Verification items for the finished model (mm, model axes). A direction names the side the tool comes from. Coordinates: 2 decimals unless noted, no trailing zeros. Write each loop counter-clockwise with the first axis right and the second up, starting at its lowest first coordinate (ties: lowest second). Pieces come first, ordered by that corner, then holes. Notation, with made-up numbers: (-32.75, -8) -> (-2.75, -8) arc R24 ccw to (-2.75, 12) -> close; hole circle Ø5 at (14, -4). An arc over 180 degrees is marked (long way). Answer in a Markdown table with one row per item.
```python
from build123d import *

# Parameters (mm, degrees)
F1_DEPTH  = 7.8
F2_R      = 6.44999
F3_R      = 2.7
F4_DEPTH  = 7.801
F5_R      = 4.2
F5_R_2    = 4.7163688055
F6_DEPTH  = 5.3
F8_DEPTH  = 10
F10_DEPTH = 5.2
F12_DEPTH = 9.8
F13_R     = 5
F14_R     = 7
F15_R     = 3
F16_R     = 3


# Not quite as in the source:
# - a fillet or chamfer is up to 0.001 mm smaller than in the source, because OpenCascade refuses the exact size


with BuildPart() as f1:
    # F0 (on Top) → F1 (new body)
    with BuildSketch(Plane.XY):
        Polygon((0, 68), (0, 12.9), (-10.05, 12.9), (-10.05, 0), (0, 0), (122, 0), (132.05, 0), (132.05, 12.9), (122, 12.9), (122, 58), (132.05, 58), (132.05, 70.9), (122, 70.9), (122, 87.4), (93.5, 87.4), (60, 68), (22.4718242228, 68), (22.4718242228, 78.05), (9.5718242228, 78.05), (9.5718242228, 68), align=None)
    extrude(amount=F1_DEPTH)

    # F2 (radius 6.45 in the source; OpenCascade refuses exactly that, so slightly less here)
    f2_edges = [f1.edges().sort_by_distance(p)[0] for p in [
        (-10.05, 0, 3.9),
        (-10.05, 12.9, 3.9),
        (9.571824, 78.05, 3.9),
        (22.471824, 78.05, 3.9),
        (132.05, 70.9, 3.9),
        (132.05, 58, 3.9),
        (132.05, 12.9, 3.9),
        (132.05, 0, 3.9),
    ]]
    fillet(f2_edges, radius=F2_R)

    # F3 (on face) → F4 (cut, through all)
    with BuildSketch(Plane.XY.offset(7.8)):
        with Locations((-3.6, 6.45)):
            Circle(F3_R)
        with Locations((16.0218242228, 71.6)):
            Circle(F3_R)
        with Locations((125.6, 64.45)):
            Circle(F3_R)
        with Locations((125.6, 6.45)):
            Circle(F3_R)
    extrude(amount=-F4_DEPTH, mode=Mode.SUBTRACT)

    # F5 (on face) → F6 (cut)
    with BuildSketch(Plane.XY.offset(7.8)):
        with Locations((-3.6, 6.45)):
            Circle(F5_R)
        with Locations((16.0218242228, 71.6)):
            Circle(F5_R)
        with Locations((125.6, 64.45)):
            Circle(F5_R_2)
        with Locations((125.6, 6.45)):
            Circle(F5_R_2)
    extrude(amount=-F6_DEPTH, mode=Mode.SUBTRACT)

    # F7 (on face) → F8 (join)
    with BuildSketch(Plane.XY.offset(7.8)):
        Polygon((5.3, 62.7), (5.3, 5.3), (116.7, 5.3), (116.7, 82.1), (94.9238653477, 82.1), (61.4238653477, 62.7), align=None)
    extrude(amount=F8_DEPTH)

    # F9 (on face) → F10 (cut)
    with BuildSketch(Plane(origin=(0, 0, 0), x_dir=(1, 0, 0), z_dir=(0, 0, -1))):
        Polygon((94.0910384462, -85.2), (119.8, -85.2), (119.8, -2.2), (2.2, -2.2), (2.2, -65.8), (60.5910384462, -65.8), align=None)
    extrude(amount=-F10_DEPTH, mode=Mode.SUBTRACT)

    # F11 (on face) → F12 (cut)
    with BuildSketch(Plane(origin=(0, 0, 5.2), x_dir=(1, 0, 0), z_dir=(0, 0, -1))):
        Polygon((114.5, -7.5), (7.5, -7.5), (7.5, -60.5), (62.0149037939, -60.5), (95.5149037939, -79.9), (114.5, -79.9), align=None)
    extrude(amount=-F12_DEPTH, mode=Mode.SUBTRACT)

    # F13
    f13_edges = [f1.edges().sort_by_distance(p)[0] for p in [
        (114.5, 79.9, 10.1),
        (119.8, 85.2, 2.6),
        (7.5, 60.5, 10.1),
        (2.2, 65.8, 2.6),
        (114.5, 7.5, 10.1),
        (7.5, 7.5, 10.1),
        (95.514904, 79.9, 10.1),
        (62.014904, 60.5, 10.1),
        (60.591038, 65.8, 2.6),
        (94.091038, 85.2, 2.6),
    ]]
    fillet(f13_edges, radius=F13_R)

    # F14
    f14_edges = [f1.edges().sort_by_distance(p)[0] for p in [
        (122, 87.4, 3.9),
        (93.5, 87.4, 3.9),
        (60, 68, 3.9),
        (61.423865, 62.7, 12.8),
        (94.923865, 82.1, 12.8),
        (116.7, 82.1, 12.8),
        (116.7, 5.3, 12.8),
        (5.3, 5.3, 12.8),
        (5.3, 62.7, 12.8),
        (0, 68, 3.9),
    ]]
    fillet(f14_edges, radius=F14_R)

    # F15
    f15_edges = [f1.edges().sort_by_distance(p)[0] for p in [
        (119.8, 2.2, 2.6),
        (2.2, 2.2, 2.6),
    ]]
    fillet(f15_edges, radius=F15_R)

    # F16
    f16_edges = [f1.edges().sort_by_distance(p)[0] for p in [
        (0, 12.9, 3.9),
        (9.571824, 68, 3.9),
        (22.471824, 68, 3.9),
        (122, 70.9, 3.9),
        (122, 58, 3.9),
        (122, 12.9, 3.9),
    ]]
    fillet(f16_edges, radius=F16_R)


solid = f1.part
```
1. Section check B-B, the plane x = 107. Record the boundary of the cut face in (y, z), plus the area to 3 significant figures.
Geometry says:
| item | result |
|---|---|
| outline | (0, 0) -> (2.2, 0) -> (2.2, 5.2) -> (7.5, 5.2) -> (7.5, 15) -> (79.9, 15) -> (79.9, 5.2) -> (85.2, 5.2) -> (85.2, 0) -> (87.4, 0) -> (87.4, 7.8) -> (82.1, 7.8) -> (82.1, 17.8) -> (5.3, 17.8) -> (5.3, 7.8) -> (0, 7.8) -> close |
| area | 309 mm^2 |
2. Section check A-A, the plane z = 9.5. Record the boundary of the cut face in (x, y), plus the area to 3 significant figures.
Geometry says:
| item | result |
|---|---|
| outline | (5.3, 12.3) arc R7 ccw to (12.3, 5.3) -> (109.7, 5.3) arc R7 ccw to (116.7, 12.3) -> (116.7, 75.1) arc R7 ccw to (109.7, 82.1) -> (96.8, 82.1) arc R7 ccw to (93.3, 81.16) -> (63.05, 63.64) arc R7 cw to (59.54, 62.7) -> (12.3, 62.7) arc R7 ccw to (5.3, 55.7) -> close; hole (7.5, 12.5) arc R5 ccw to (12.5, 7.5) -> (109.5, 7.5) arc R5 ccw to (114.5, 12.5) -> (114.5, 74.9) arc R5 ccw to (109.5, 79.9) -> (96.86, 79.9) arc R5 ccw to (94.35, 79.23) -> (63.18, 61.17) arc R5 cw to (60.67, 60.5) -> (12.5, 60.5) arc R5 ccw to (7.5, 55.5) -> close |
| area | 757 mm^2 |
3. Tool access check on faces 1 (the cylindrical face through (114.6, 7.3, 12.9)), 2 (the flat face through (0, 39, 4)), 3 (the cylindrical face through (118.94, 3.1, 2.64)), 4 (the cylindrical face through (122.9, 13.76, 3.95)). Record the directions out of +Z, -Z, +X, -X, +Y, -Y that give a thin tool (end or side, any length) a straight path to the whole face; none if there is none.
Geometry says:
| item | result |
|---|---|
| face 1 | +Z, +X, -Y |
| face 2 | +Z, -Z, -X, +Y |
| face 3 | -Z |
| face 4 | +Z, -Z, +X |
4. Thickness scan on line 1 (X direction, y = 22.5, z = 9.5); line 2 (Y direction, x = 48, z = 3.25); line 3 (Y direction, x = 100, z = 8.75). Record the ranges inside material, lowest first. Write a range as from..to.
Geometry says:
| item | result |
|---|---|
| line 1 | 5.3..7.5, 114.5..116.7 |
| line 2 | 0..2.2, 65.8..68 |
| line 3 | 5.3..7.5, 79.9..82.1 |
5. Depth check by flat-ended pin: P1, Ø1.5, axis at x = 75.5, y = 12.5, coming from the -Z side; P2, Ø8, axis at x = 82, z = 10.5, coming from the -Y side; P3, Ø7, axis at x = 125.6, y = 64.45, coming from the +Z side; P4, Ø3, axis at x = 105.5, z = 14, coming from the +Y side. Enter the tip coordinate at first touch or a pass-through.
Geometry says:
| item | result |
|---|---|
| P1 | z = 15 |
| P2 | y = 0 |
| P3 | z = 2.5 |
| P4 | y = 82.1 |
6. Section check C-C, the plane x = 41. Record the boundary of the cut face in (y, z), plus the area to 3 significant figures.
Geometry says:
| item | result |
|---|---|
| outline | (0, 0) -> (2.2, 0) -> (2.2, 5.2) -> (7.5, 5.2) -> (7.5, 15) -> (60.5, 15) -> (60.5, 5.2) -> (65.8, 5.2) -> (65.8, 0) -> (68, 0) -> (68, 7.8) -> (62.7, 7.8) -> (62.7, 17.8) -> (5.3, 17.8) -> (5.3, 7.8) -> (0, 7.8) -> close |
| area | 254 mm^2 |
